The model under review builds one solid part; all positions refer to its coordinate system, in mm. Face numbers are marked on the shaded views. A direction names the side the tool comes from. Coordinates: 2 decimals unless noted, no trailing zeros. Write each loop counter-clockwise with the first axis right and the second up, starting at its lowest first coordinate (ties: lowest second). Pieces come first, ordered by that corner, then holes. Notation, with made-up numbers: (-1, -12) - (58, -12) arc R17 ccw to (58, 6) - close; hole circle Ø10 at (-39.5, -37). An arc over 180 degrees is marked (long way). Put each result on its own line as item: value. Start each with the question number.
Item 1: Consider section C-C on x = 2. Give the boundary of the cut face in (y, z) (3 decimals), then the cut area to 3 significant figures.
Item 2: For pin 1 (10 mm diameter, centred on y = 44.5, z = 14.5, fed in from -X); pin 2 (6.5 mm diameter, centred on y = 2.5, z = 16.5, fed in from +X); pin 3 (8 mm diameter, centred on x = -70, z = 20, fed in from +Y); pin 4 (8 mm diameter, centred on x = -62.5, y = 40, fed in from -Z), all flat-tipped, find the tip position at first contact; note any pin that passes through.
Item 3: To check wall thickness, follow L1, parallel to X at y = 1.95, z = 5; L2, parallel to X at y = 4.1, z = 5; L3, parallel to Z at x = 66.5, y = 5. State the ranges of each line that lie inside material, in increasing order. Write a range as [from, to].
Item 4: Machinability: for the marked faces 1, 2, 3, 4 and 5, which of the approach directions +Z, -Z, +X, -X, +Y, -Y give a long, thin tool a straight path to every point of the face, cutting with its end or side? Answer none if there is none.
Item 5: Consider section A-A on y = 15. Give the boundary of the cut face in (x, z), then the cut area to 3 significant figures.
Item 6: Consider section B-B on x = -17. Give the boundary of the cut face in (y, z), then the cut area to 3 significant figures.
Item 7: Mouldability with a two-part tool opening along Y and no side actions: class the marked faces 6, 7, 8 and 9 as pulls with the +Y half, pulls with the -Y half, needs draft (parallel to the pull), parting line crosses it, or undercut.
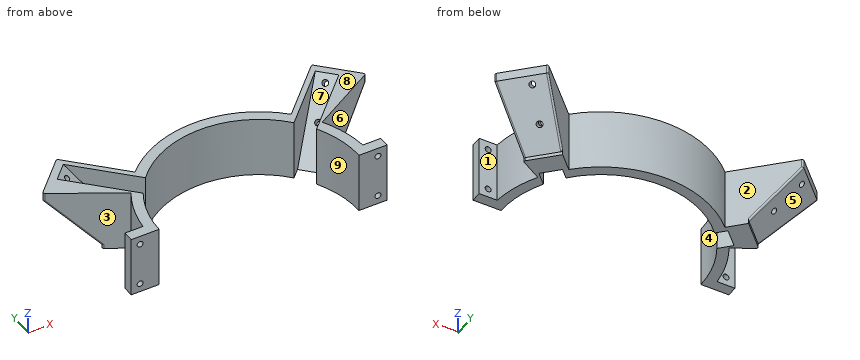
```python
from build123d import *

# Parameters (mm, degrees)
EXTRUDE_1_DEPTH     = 35
EXTRUDE_START       = -35
EXTRUDE_2_DEPTH     = 35
CUT_EXTRUDE_1_DEPTH = 123.873256546
SKETCH_4_W          = 12
SKETCH_4_H          = 35
CUT_EXTRUDE_4_DEPTH = 165.71136734
FILLET_1_R          = 1
FILLET_2_R          = 1
SKETCH_5_W          = 13
SKETCH_5_H          = 6
EXTRUDE_4_DEPTH     = 35


# Read off the part's stored shape, not the designer's step: M3 すきま穴1, M3 すきま穴2
with BuildPart() as part:
    # ｽｹｯﾁ1 → ﾎﾞｽ - 押し出し1 (new body)
    with BuildSketch(Plane.XY):
        with BuildLine():
            Line((57.15, 0), (63.15, 0))
            ThreePointArc((63.15, 0), (0, 63.15), (-63.15, 0))
            Line((-63.15, 0), (-57.15, 0))
            ThreePointArc((-57.15, 0), (0, 57.15), (57.15, 0))
        make_face()
    extrude(amount=EXTRUDE_1_DEPTH)

    # ｽｹｯﾁ2 → ﾎﾞｽ - 押し出し2 (add)
    with BuildSketch(Plane.XY.offset(35).offset(EXTRUDE_START)):
        with BuildLine():
            Line((-44.653793232, 44.653793232), (-72.938064479, 72.938064479))
            Line((-72.938064479, 72.938064479), (-92.481759954, 53.394369005))
            Line((-92.481759954, 53.394369005), (-54.689504249, 31.575))
            ThreePointArc((-54.689504249, 31.575), (-50.100263439, 38.443284242), (-44.653793232, 44.653793232))
        make_face()
    extrude_2 = extrude(amount=EXTRUDE_2_DEPTH)

    # ｽｹｯﾁ3 → ｶｯﾄ - 押し出し1 (cut, through all)
    with BuildSketch(Plane(origin=(0, 0, 0), x_dir=(0, 0, -1), z_dir=(0.7071067811865461, 0.7071067811865489, 0))):
        Polygon((-30, 103.15), (-2, 75.15), (0, 75.15), (0, 103.15), align=None)
    cut_extrude_1 = extrude(amount=-CUT_EXTRUDE_1_DEPTH, mode=Mode.SUBTRACT)

    # ﾐﾗｰ1: ﾎﾞｽ - 押し出し2, ｶｯﾄ - 押し出し1 across plane
    add(extrude_2.mirror(Plane(origin=(0, 0, 0), x_dir=(0, 0, 1), z_dir=(1, 0, 0))))
    add(cut_extrude_1.mirror(Plane(origin=(0, 0, 0), x_dir=(0, 0, 1), z_dir=(1, 0, 0))), mode=Mode.SUBTRACT)

    # ｽｹｯﾁ4 → ｶｯﾄ - 押し出し4 (cut, through all)
    with BuildSketch(Plane(origin=(-48.84340091, 48.84340091, 69.075), x_dir=(-0.707106781186546, -0.707106781186549, 0), z_dir=(0.5000000000000019, -0.4999999999999998, -0.7071067811865465))):
        with Locations((9, 27.689327138)):
            Rectangle(SKETCH_4_W, SKETCH_4_H)
    cut_extrude_4 = extrude(amount=CUT_EXTRUDE_4_DEPTH, mode=Mode.SUBTRACT)

    # ﾌｨﾚｯﾄ1
    fillet_1_edges = [part.edges().sort_by_distance(p)[0] for p in [
        (-72.938064479, 72.938064479, 32.5),
        (-92.481759954, 53.394369005, 32.5),
        (-67.377646733, 38.900502479, 1),
        (-79.929703344, 46.147435742, 16),
        (-63.038569543, 63.038569543, 16),
    ]]
    fillet(fillet_1_edges, radius=FILLET_1_R)

    # ﾐﾗｰ3: ｶｯﾄ - 押し出し4 across plane
    add(cut_extrude_4.mirror(Plane(origin=(0, 0, 0), x_dir=(0, 0, 1), z_dir=(1, 0, 0))), mode=Mode.SUBTRACT)

    # ﾌｨﾚｯﾄ2
    fillet_2_edges = [part.edges().sort_by_distance(p)[0] for p in [
        (72.938064479, 72.938064479, 32.5),
        (92.481759954, 53.394369005, 32.5),
        (63.038569543, 63.038569543, 16),
        (79.929703344, 46.147435742, 16),
        (67.377646733, 38.900502479, 1),
    ]]
    fillet(fillet_2_edges, radius=FILLET_2_R)

    # ｽｹｯﾁ5 → ﾎﾞｽ - 押し出し4 (add)
    with BuildSketch(Plane.XY.offset(35)):
        with Locations((-66.65, 3)):
            Rectangle(SKETCH_5_W, SKETCH_5_H)
        with Locations((66.65, 3)):
            Rectangle(SKETCH_5_W, SKETCH_5_H)
    extrude(amount=-EXTRUDE_4_DEPTH)

    # M3 すきま穴1 outline → M3 すきま穴1 (revolve, cut)
    with BuildSketch(Plane(origin=(68.007159089, 0, 30), x_dir=(1, 0, 0), z_dir=(0, 0, 1))):
        Polygon((0, 0), (1.7, 0), (1.7, 5.97124079), (1.725, 6), (0, 6), align=None)
    revolve(axis=Axis((68.007159089, 0, 30), (0, 1, 0)), mode=Mode.SUBTRACT)

    # Hole Wizard M3 _1 2 outline → Hole Wizard M3 _1 2 (revolve, cut)
    with BuildSketch(Plane(origin=(68.007159089, 0, 5), x_dir=(1, 0, 0), z_dir=(0, 0, 1))):
        Polygon((0, 0), (1.7, 0), (1.7, 5.97124079), (1.725, 6), (0, 6), align=None)
    revolve(axis=Axis((68.007159089, 0, 5), (0, 1, 0)), mode=Mode.SUBTRACT)

    # Hole Wizard M3 _1 3 outline → Hole Wizard M3 _1 3 (revolve, cut)
    with BuildSketch(Plane(origin=(-68.007159089, 0, 30), x_dir=(1, 0, 0), z_dir=(0, 0, 1))):
        Polygon((0, 0), (1.7, 0), (1.7, 5.97124079), (1.725, 6), (0, 6), align=None)
    revolve(axis=Axis((-68.007159089, 0, 30), (0, 1, 0)), mode=Mode.SUBTRACT)

    # Hole Wizard M3 _1 4 outline → Hole Wizard M3 _1 4 (revolve, cut)
    with BuildSketch(Plane(origin=(-68.007159089, 0, 5), x_dir=(1, 0, 0), z_dir=(0, 0, 1))):
        Polygon((0, 0), (1.7, 0), (1.7, 5.97124079), (1.725, 6), (0, 6), align=None)
    revolve(axis=Axis((-68.007159089, 0, 5), (0, 1, 0)), mode=Mode.SUBTRACT)

    # M3 すきま穴2 outline → M3 すきま穴2 (revolve, cut)
    with BuildSketch(Plane(origin=(-41.207361941, 28.47943988, 49.276010127), x_dir=(0.8660254037844382, 0.28867513459481287, -0.4082482904638642), z_dir=(0, -0.8164965809277269, -0.5773502691896247))):
        Polygon((0, -51.724861044), (1.7, -51.724861044), (1.7, -45.218086348), (1.725, -45.189327138), (0, -45.189327138), align=None)
    hole_wizard_m3_2 = revolve(axis=Axis((-41.207361941, 28.47943988, 49.276010127), (0.500000000000001, -0.49999999999999883, 0.7071067811865479)), mode=Mode.SUBTRACT)

    # Hole Wizard M3 _2 2 outline → Hole Wizard M3 _2 2 (revolve, cut)
    with BuildSketch(Plane(origin=(-51.207361941, 38.47943988, 63.418145751), x_dir=(0.8660254037844382, 0.28867513459481287, -0.4082482904638642), z_dir=(0, -0.8164965809277269, -0.5773502691896247))):
        Polygon((0, -51.724861044), (1.7, -51.724861044), (1.7, -45.218086348), (1.725, -45.189327138), (0, -45.189327138), align=None)
    hole_wizard_m3_2_2 = revolve(axis=Axis((-51.207361941, 38.47943988, 63.418145751), (0.500000000000001, -0.49999999999999883, 0.7071067811865479)), mode=Mode.SUBTRACT)

    # ﾐﾗｰ5: M3 すきま穴2, Hole Wizard M3 _2 2 across plane
    add(hole_wizard_m3_2.mirror(Plane(origin=(0, 0, 0), x_dir=(0, 0, 1), z_dir=(1, 0, 0))), mode=Mode.SUBTRACT)
    add(hole_wizard_m3_2_2.mirror(Plane(origin=(0, 0, 0), x_dir=(0, 0, 1), z_dir=(1, 0, 0))), mode=Mode.SUBTRACT)


solid = part.part
```
Report:
1. outline: (57.115, 0) - (63.118, 0) - (63.118, 35) - (57.115, 35) - close
1. area: 210 mm²
2. pin 1: x = -81.48
2. pin 2: x = 73.15
2. pin 3: y = 68.09
2. pin 4: z = 0
3. L1: [-73.15, -69.71], [-66.31, -57.12], [57.12, 66.31], [69.71, 73.15]
3. L2: [-73.15, -69.71], [-66.31, -57], [57, 66.31], [69.71, 73.15]
3. L3: [0, 4.21], [5.79, 29.21], [30.79, 35]
4. face 1: +Z, -Z, +X
4. face 2: +Z, -Z, +Y
4. face 3: +Z, -Z, -X
4. face 4: +Z, -Z, -Y
4. face 5: -Z, -X, +Y
5. outline: (-61.34, 0) - (-55.15, 0) - (-55.15, 35) - (-61.34, 35) - close; (55.15, 0) - (61.34, 0) - (61.34, 35) - (55.15, 35) - close
5. area: 434 mm²
6. outline: (54.56, 0) - (60.82, 0) - (60.82, 35) - (54.56, 35) - close
6. area: 219 mm²
7. face 6: undercut
7. face 7: undercut
7. face 8: needs draft
7. face 9: pulls with the -Y half
